For this review, take the finished solid that the model builds, in its own axes (mm). A direction names the side the tool comes from. Round coordinates to 2 decimals unless told otherwise and drop trailing zeros. Write each loop counter-clockwise with the first axis right and the second up, starting at its lowest first coordinate (ties: lowest second). Pieces come first, ordered by that corner, then holes.
from build123d import *

# Parameters (mm, degrees)
F0_W     = 127
F0_H     = 88.9
F1_DEPTH = 3
F2_W     = 127
F2_H     = 88.9
F2_W_2   = 121
F2_H_2   = 82.9
F3_DEPTH = 114.3
F4_R     = 5


with BuildPart() as f1:
    # F0 (on Top) → F1 (new body)
    with BuildSketch(Plane.XY):
        Rectangle(F0_W, F0_H)
    extrude(amount=F1_DEPTH)

    # F2 (on face) → F3 (join)
    with BuildSketch(Plane.XY.offset(3)):
        Rectangle(F2_W, F2_H)
        Rectangle(F2_W_2, F2_H_2, mode=Mode.SUBTRACT)
    extrude(amount=F3_DEPTH)

    # F4
    f4_edges = [f1.edges().sort_by_distance(p)[0] for p in [
        (0, -41.45, 3),
        (-60.5, 0, 3),
        (-60.5, -41.45, 60.15),
        (-60.5, 41.45, 60.15),
        (0, 41.45, 3),
        (60.5, 41.45, 60.15),
        (60.5, 0, 3),
        (60.5, -41.45, 60.15),
        (63.5, -44.45, 58.65),
        (63.5, 44.45, 58.65),
        (-63.5, 44.45, 58.65),
        (-63.5, -44.45, 58.65),
    ]]
    fillet(f4_edges, radius=F4_R)


solid = f1.part
(1) We need section A-A, the plane z = 110. Give the boundary of the cut face in (x, y).
Geometry check:
outline: (-63.5, -39.45) arc R5 ccw to (-58.5, -44.45) - (58.5, -44.45) arc R5 ccw to (63.5, -39.45) - (63.5, 39.45) arc R5 ccw to (58.5, 44.45) - (-58.5, 44.45) arc R5 ccw to (-63.5, 39.45) - close; hole (-60.5, -36.45) arc R5 ccw to (-55.5, -41.45) - (55.5, -41.45) arc R5 ccw to (60.5, -36.45) - (60.5, 36.45) arc R5 ccw to (55.5, 41.45) - (-55.5, 41.45) arc R5 ccw to (-60.5, 36.45) - close
(2) For pin 1 Ø1 at (x, y) = (37.5, 4.5) entering from +Z, flat-tipped, find the tip position at first contact; note if it passes through.
Geometry check:
pin 1: stops at z = 3
(3) For faces 4 (the face through (63.5, -1, 58)), 5 (the face through (-59.07, 39.95, 63.42)), list the 3-axis set-ups (+Z, -Z, +X, -X, +Y, -Y) from which the entire face can be reached by the end or side of a thin tool; tool diameter is ignored.
Geometry check:
face 4: +Z, -Z, +X, +Y, -Y
face 5: +Z
(4) We need section C-C, the plane y = -7.5. Give the boundary of the cut face in (x, z), and give its area (3 significant figures).
Geometry check:
outline: (-63.5, 0) - (63.5, 0) - (63.5, 117.3) - (60.5, 117.3) - (60.5, 8) arc R5 cw to (55.5, 3) - (-55.5, 3) arc R5 cw to (-60.5, 8) - (-60.5, 117.3) - (-63.5, 117.3) - close
area: 1,080 mm2
(5) For line 1 along X through (y, z) = (-18, 14); line 2 along Y through (x, z) = (19, 37); line 3 along Z through (x, y) = (-4.5, -12.5), list the stretches that pass through material, from the lowest coordinate up.
Geometry check:
line 1: x = -63.5 to -60.5, 60.5 to 63.5
line 2: y = -44.45 to -41.45, 41.45 to 44.45
line 3: z = 0 to 3
(6) Mouldability with a two-part tool opening along X and no side actions: class faces 1 (the face through (-62.07, 42.95, 57.83)), 2 (the face through (-60.5, -1, 62)), 3 (the face through (62.07, 42.95, 57.83)) as pulls with the +X half, pulls with the -X half, needs draft (parallel to the pull), parting line crosses it, or undercut.
Geometry check:
face 1: pulls with the -X half
face 2: undercut
face 3: pulls with the +X half
(7) We need section B-B, the plane x = -12. Give the boundary of the cut face in (y, z), and give its area (3 significant figures).
Geometry check:
outline: (-44.45, 0) - (44.45, 0) - (44.45, 117.3) - (41.45, 117.3) - (41.45, 8) arc R5 cw to (36.45, 3) - (-36.45, 3) arc R5 cw to (-41.45, 8) - (-41.45, 117.3) - (-44.45, 117.3) - close
area: 963 mm2
